Here's how the part is built. I have some questions about the finished solid (model axes, mm). A direction names the side the tool comes from. Give positions to 0.01 mm unless a question says otherwise; leave off trailing zeros. Write each loop counter-clockwise with the first axis right and the second up, starting at its lowest first coordinate (ties: lowest second). Pieces come first, ordered by that corner, then holes. Notation, with made-up numbers: (31.25, 74) - (77.25, 74) arc R22 cw to (77.25, 83) - close; hole circle Ø11 at (50.5, 68.25). An arc over 180 degrees is marked (long way). Write each question's results on one line, items separated by ' | '. Start each with the question number.
Item 1: Will these pins go through, and if not, where does the flat tip stop? P1, Ø6.5, axis at x = -5, y = -19, coming from the +Z side; P2, Ø1.2, axis at y = -16.5, z = -16.5, coming from the +X side; P3, Ø2, axis at y = -17, z = -8.5, coming from the +X side.
Item 2: We'd pull the mould along X, two halves only. Please class faces 4 (the flat face through (-7, -7.675, -9)), 5 (the flat face through (-7, -17, -15.9)), 6 (the flat face through (-21.709, -17, -9)), 7 (the flat face through (4.791, -21, -8)): +X half, -X half, draft (parallel to the pull), parting line (faces both ways), or undercut.
Item 3: Suppose I cut it at B-B on x = -13. List the corners of the cut face in (y, z) for me.
Item 4: Please list where these lines run through material, in increasing order: line 1 along X through (y, z) = (-11.5, -2.5); line 2 along Y through (x, z) = (-11.25, -1.25); line 3 along Z through (x, y) = (2.25, -12).
Item 5: Suppose I cut it at A-A on z = -8. List the corners of the cut face in (x, y) for me, then the cut area to 3 significant figures.
Item 6: Suppose I cut it at C-C on y = -13.5. List the corners of the cut face in (x, z) for me, then the cut area to 3 significant figures.
Item 7: Which directions (+Z, -Z, +X, -X, +Y, -Y) give clear straight access to the entire face, cutting with the end or side of a thin tool? Please do faces 1 (the flat face through (-7, -10, 0)), 2 (the flat face through (6, -18.925, -9)), 3 (the flat face through (-7, -23.175, -8)).
```python
from build123d import *

# Parameters (mm, degrees)
F0_W     = 24
F0_H     = 13
F1_DEPTH = 15.9
F2_T     = 2.5
F3_W     = 4.5
F3_H     = 2.5
F4_DEPTH = 2.5


with BuildPart() as f1:
    # F0 (on Top) → F1 (new body)
    with BuildSketch(Plane.XY):
        with Locations((-7.2094501108, -16.6747012585)):
            Rectangle(F0_W, F0_H)
    extrude(amount=-F1_DEPTH)

    # F2
    f2_openings = [f1.faces().sort_by_distance(p)[0] for p in [
        (-7.20945, -16.674701, 0),
    ]]
    offset(amount=F2_T, openings=f2_openings, kind=Kind.INTERSECTION)

    # F3 (on face) → F4 (cut)
    with BuildSketch(Plane.YZ.offset(7.2905498892)):
        Polygon((-14.4247012585, 0), (-16.6747012585, 0), (-18.9247012585, 0), (-18.9247012585, -15.9), (-14.4247012585, -15.9), align=None)
        with Locations((-16.6747012585, -17.15)):
            Rectangle(F3_W, F3_H)
    extrude(amount=-F4_DEPTH, mode=Mode.SUBTRACT)


solid = f1.part
```
Checked values:
1) P1: stops at z = -15.9 | P2: stops at x = 4.79 | P3: stops at x = -19.21
2) face 4: draft | face 5: undercut | face 6: -X half | face 7: undercut
3) outline: (-25.67, -18.4) - (-7.67, -18.4) - (-7.67, 0) - (-10.17, 0) - (-10.17, -15.9) - (-23.17, -15.9) - (-23.17, 0) - (-25.67, 0) - close
4) line 1: x = -21.71 to -19.21, 4.79 to 7.29 | line 2: y = -25.67 to -23.17, -10.17 to -7.67 | line 3: z = -18.4 to -15.9
5) outline: (-21.71, -25.67) - (7.29, -25.67) - (7.29, -18.92) - (4.79, -18.92) - (4.79, -23.17) - (-19.21, -23.17) - (-19.21, -10.17) - (4.79, -10.17) - (4.79, -14.42) - (7.29, -14.42) - (7.29, -7.67) - (-21.71, -7.67) - close | area: 199 mm^2
6) outline: (-21.71, -18.4) - (7.29, -18.4) - (7.29, 0) - (4.79, 0) - (4.79, -15.9) - (-19.21, -15.9) - (-19.21, 0) - (-21.71, 0) - close | area: 152 mm^2
7) face 1: +Z, +X, -X, +Y, -Y | face 2: +Z, -Z, +X | face 3: +Z
